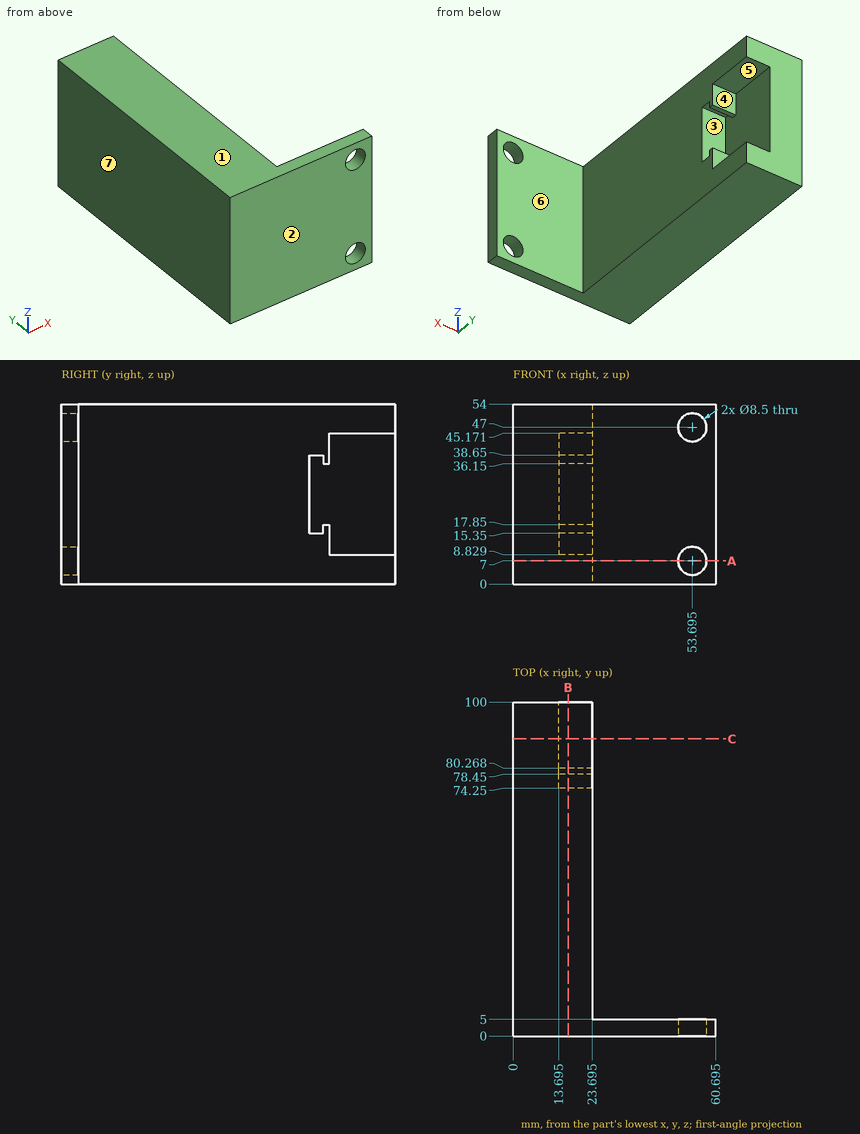
Here's the drawing with two shaded views (mm, measured from the low corner). I have some questions. A direction names the side the tool comes from. Give positions to 0.01 mm unless a question says otherwise; leave off trailing zeros. Loops run counter-clockwise (first coordinate to the right, second up) from the corner with the lowest first, then second, coordinate; pieces in that order, holes last. Notation, with made-up numbers: M 6.5,-0.75 L 25.5,-0.75 A12 cw 25.5,15.25 Z; hole C -25,27.5 d10. An arc over 180 degrees is marked long. Use one line per item in the form item = value. Start each with the question number.
Q1. If we section it at B-B (x = 16.5): Write out the boundary of the cut face in (y, z), then the cut area to 3 significant figures.
Q2. Thinking about a two-plate mould opening in Y: for the marked faces 1, 2, 3 and 4, which applies, +Y half, -Y half, draft (parallel to the pull), parting line (faces both ways), or undercut?
Q3. I need wall thicknesses on line 1 along X through (y, z) = (1, 7) (1 decimal); line 2 along X through (y, z) = (43, 32) (1 decimal); line 3 along Y through (x, z) = (57.5, 25). Which ranges of each line are inside material? Lowest first, please.
Q4. If we section it at A-A (z = 7): Write out the boundary of the cut face in (x, y) (1 decimal), then the cut area to 3 significant figures.
Q5. Which directions (+Z, -Z, +X, -X, +Y, -Y) give clear straight access to the entire face, cutting with the end or side of a thin tool? Please do the marked faces 5, 6 and 7.
Q6. Will these pins go through, and if not, where does the flat tip stop? pin 1 Ø11 at (x, z) = (53.69, 7) entering from +Y; pin 2 Ø12 at (x, y) = (35.5, 34) entering from +Z; pin 3 Ø12 at (y, z) = (79, 17.5) entering from +X (1 decimal).
Q7. If we section it at C-C (y = 89): Write out the boundary of the cut face in (x, z) (1 decimal), then the cut area to 3 significant figures.
Taken from the geometry:
q1.outline = M 0,0 L 100,0 L 100,8.83 L 80.27,8.83 L 80.27,17.85 L 78.45,17.85 L 78.45,15.35 L 74.25,15.35 L 74.25,38.65 L 78.45,38.65 L 78.45,36.15 L 80.27,36.15 L 80.27,45.17 L 100,45.17 L 100,54 L 0,54 Z
q1.area = 4,550 mm^2
q2.face_1 = draft
q2.face_2 = -Y half
q2.face_3 = undercut
q2.face_4 = +Y half
q3.line_1 = 0 to 49.4, 57.9 to 60.7
q3.line_2 = 0 to 23.7
q3.line_3 = 0 to 5
q4.outline = M 0,0 L 49.4,0 L 49.4,5 L 23.7,5 L 23.7,100 L 0,100 Z; M 57.9,0 L 60.7,0 L 60.7,5 L 57.9,5 Z
q4.area = 2,510 mm^2
q5.face_5 = +X, +Y
q5.face_6 = +Z, -Z, +X, +Y
q5.face_7 = +Z, -Z, -X, +Y, -Y
q6.pin_1 = 5
q6.pin_2 = through
q6.pin_3 = 23.7
q7.outline = M 0,0 L 23.7,0 L 23.7,8.8 L 13.7,8.8 L 13.7,45.2 L 23.7,45.2 L 23.7,54 L 0,54 Z
q7.area = 916 mm^2
